```python
from build123d import *

# Parameters (mm, degrees)
SKETCH1_W           = 9
SKETCH1_H           = 9
SKETCH1_W_2         = 3
SKETCH1_H_2         = 1.5
BOSS_EXTRUDE1_DEPTH = 0.5
FILLET1_R           = 10
FILLET3_R           = 1


with BuildPart() as part:
    # Sketch1 → Boss-Extrude1 (new, symmetric)
    with BuildSketch(Plane.XY):
        with BuildLine():
            Line((-200, 10), (-200, 20))
            Line((-200, 20), (-12.686273665, 20))
            ThreePointArc((-12.686273665, 20), (-6.83279553, 18.787212337), (-1.943060243, 15.348528137))
            Line((-1.943060243, 15.348528137), (0, 10))
            Line((0, 10), (0, 0))
            Line((0, 0), (-10, 0))
            Line((-10, 0), (-200, 0))
            Line((-200, 0), (-200, 10))
        make_face()
        Polygon((-180.8, 11), (-180.8, 6), (-160.8, 6), align=None, mode=Mode.SUBTRACT)
        with Locations((-190.3, 10)):
            Rectangle(SKETCH1_W, SKETCH1_H, mode=Mode.SUBTRACT)
        Polygon((-154.8, 7.076941016), (-154.8, 12.076941016), (-174.8, 12.076941016), align=None, mode=Mode.SUBTRACT)
        Polygon((-130.8, 6), (-110.8, 11), (-110.8, 6), align=None, mode=Mode.SUBTRACT)
        Polygon((-136.8, 7.076941016), (-136.8, 12.076941016), (-116.8, 12.076941016), align=None, mode=Mode.SUBTRACT)
        with BuildLine():
            Line((-95.102943725, 12.697056275), (-89.021825407, 6.615937957))
            ThreePointArc((-89.021825407, 6.615937957), (-89.021825407, 4.918881682), (-90.718881682, 4.918881682))
            Line((-90.718881682, 4.918881682), (-96.8, 11))
            ThreePointArc((-96.8, 11), (-96.8, 12.697056275), (-95.102943725, 12.697056275))
        make_face(mode=Mode.SUBTRACT)
        with BuildLine():
            Line((-93.794617613, 16.197056275), (-89.127712857, 11.530151519))
            ThreePointArc((-89.127712857, 11.530151519), (-89.127712857, 9.833095244), (-90.824769132, 9.833095244))
            Line((-90.824769132, 9.833095244), (-95.491673888, 14.5))
            ThreePointArc((-95.491673888, 14.5), (-95.491673888, 16.197056275), (-93.794617613, 16.197056275))
        make_face(mode=Mode.SUBTRACT)
        with Locations((-89.794617613, 18.25)):
            Rectangle(SKETCH1_W_2, SKETCH1_H_2, mode=Mode.SUBTRACT)
        with Locations((-62.460808101, 18.25)):
            Rectangle(SKETCH1_W_2, SKETCH1_H_2, mode=Mode.SUBTRACT)
        with BuildLine():
            Line((-58.460808101, 16.197056275), (-63.127712857, 11.530151519))
            ThreePointArc((-63.127712857, 11.530151519), (-63.127712857, 9.833095244), (-61.430656582, 9.833095244))
            Line((-61.430656582, 9.833095244), (-56.763751827, 14.5))
            ThreePointArc((-56.763751827, 14.5), (-56.763751827, 16.197056275), (-58.460808101, 16.197056275))
        make_face(mode=Mode.SUBTRACT)
        with BuildLine():
            Line((-57.152481989, 12.697056275), (-63.233600308, 6.615937957))
            ThreePointArc((-63.233600308, 6.615937957), (-63.233600308, 4.918881682), (-61.536544033, 4.918881682))
            Line((-61.536544033, 4.918881682), (-55.455425715, 11))
            ThreePointArc((-55.455425715, 11), (-55.455425715, 12.697056275), (-57.152481989, 12.697056275))
        make_face(mode=Mode.SUBTRACT)
        Polygon((-25.2, 12.076941016), (-45.2, 7.076941016), (-45.2, 12.076941016), align=None, mode=Mode.SUBTRACT)
        Polygon((-39.2, 6), (-19.2, 11), (-19.2, 6), align=None, mode=Mode.SUBTRACT)
        with BuildLine():
            Line((-17.321963125, 16.390064684), (-14.260022427, 12.437278431))
            ThreePointArc((-14.260022427, 12.437278431), (-14.47382536, 10.753743963), (-16.157359828, 10.967546896))
            Line((-16.157359828, 10.967546896), (-19.219300527, 14.920333149))
            ThreePointArc((-19.219300527, 14.920333149), (-19.005497594, 16.603867617), (-17.321963125, 16.390064684))
        make_face(mode=Mode.SUBTRACT)
        with BuildLine():
            Line((-12.321963125, 14.907009966), (-9.260022427, 10.954223713))
            ThreePointArc((-9.260022427, 10.954223713), (-9.47382536, 9.270689245), (-11.157359828, 9.484492178))
            Line((-11.157359828, 9.484492178), (-14.219300527, 13.437278431))
            ThreePointArc((-14.219300527, 13.437278431), (-14.005497594, 15.120812899), (-12.321963125, 14.907009966))
        make_face(mode=Mode.SUBTRACT)
        with BuildLine():
            Line((-7.321963125, 15.376741501), (-4.260022427, 11.423955248))
            ThreePointArc((-4.260022427, 11.423955248), (-4.47382536, 9.74042078), (-6.157359828, 9.954223713))
            Line((-6.157359828, 9.954223713), (-9.219300527, 13.907009966))
            ThreePointArc((-9.219300527, 13.907009966), (-9.005497594, 15.590544434), (-7.321963125, 15.376741501))
        make_face(mode=Mode.SUBTRACT)
    extrude(amount=BOSS_EXTRUDE1_DEPTH, both=True)

    # Fillet1
    fillet1_edges = [part.edges().sort_by_distance(p)[0] for p in [
        (0, 10, 0),
        (-1.943060243, 15.348528137, 0),
    ]]
    fillet(fillet1_edges, radius=FILLET1_R)

    # Fillet3
    fillet3_edges = [part.edges().sort_by_distance(p)[0] for p in [
        (-200, 20, 0),
        (-154.8, 7.076941016, 0),
        (-154.8, 12.076941016, 0),
        (-180.8, 11, 0),
        (-180.8, 6, 0),
        (-194.8, 14.5, 0),
        (-194.8, 5.5, 0),
        (-185.8, 5.5, 0),
        (-185.8, 14.5, 0),
        (-110.8, 6, 0),
        (-110.8, 11, 0),
        (-136.8, 7.076941016, 0),
        (-136.8, 12.076941016, 0),
        (-45.2, 12.076941016, 0),
        (-45.2, 7.076941016, 0),
        (-19.2, 6, 0),
        (-19.2, 11, 0),
    ]]
    fillet(fillet3_edges, radius=FILLET3_R)


solid = part.part
```
The listing builds one solid part. Answer for the finished solid, in the listing's coordinates (mm). A direction names the side the tool comes from. Give positions to 0.01 mm unless a question says otherwise; leave off trailing zeros. Put each result on its own line as item: value. Start each with the question number.
Item 1: Flat-ended cylindrical pins translate along their axes: P1, Ø0.5, axis at y = 18, z = 0, coming from the +X side; P2, Ø0.5, axis at y = 9.5, z = 0, coming from the +X side. Find the tip coordinate at first contact, or state that the pin passes through.
Item 2: The part is cut by section A-A, the plane z = -0.35. State how many separate pieces and enclosed holes the cut face has, and give its area (3 significant figures).
Item 3: Which of the six approach directions +Z, -Z, +X, -X, +Y, -Y give full straight-line access (tool end or side, diameter ignored) to faces 4 (the face through (-99, 10, -0.5)), 5 (the face through (-5.812, 13.428, 0.007))?
Item 4: Find the intervals of material crossed by line 1 along Y through (x, z) = (-166, 0.05); line 2 along Y through (x, z) = (-115.5, 0.4) (3 decimals); line 3 along Y through (x, z) = (-30, -0.4), in increasing order.
Item 5: For a pull along Y with two mould halves and no side action, classify faces 1 (the face through (-2.824, 15.918, -0.007)), 2 (the face through (-99, 10, 0.5)), 3 (the face through (-12.667, 11.433, 0.007)) as +Y half, -Y half, draft (parallel to the pull), parting line (faces both ways), or undercut.
Answer key:
1. P1: stops at x = -4.89
1. P2: stops at x = -0.05
2. separate pieces: 1
2. enclosed holes: 16
2. area: 3,440 mm²
3. face 4: -Z, +X, -X, +Y, -Y
3. face 5: +Z, -Z
4. line 1: y = 0 to 6, 7.3 to 9.88, 12.08 to 20
4. line 2: y = 0 to 6, 9.825 to 20
4. line 3: y = 0 to 6, 8.3 to 10.88, 12.08 to 20
5. face 1: +Y half
5. face 2: draft
5. face 3: undercut
